Part print with two shaded views. Sizes in mm from the minimum x, y, z corner. A direction names the side the tool comes from. Give positions to 0.01 mm unless a question says otherwise; leave off trailing zeros. Write each loop counter-clockwise with the first axis right and the second up, starting at its lowest first coordinate (ties: lowest second). Pieces come first, ordered by that corner, then holes.
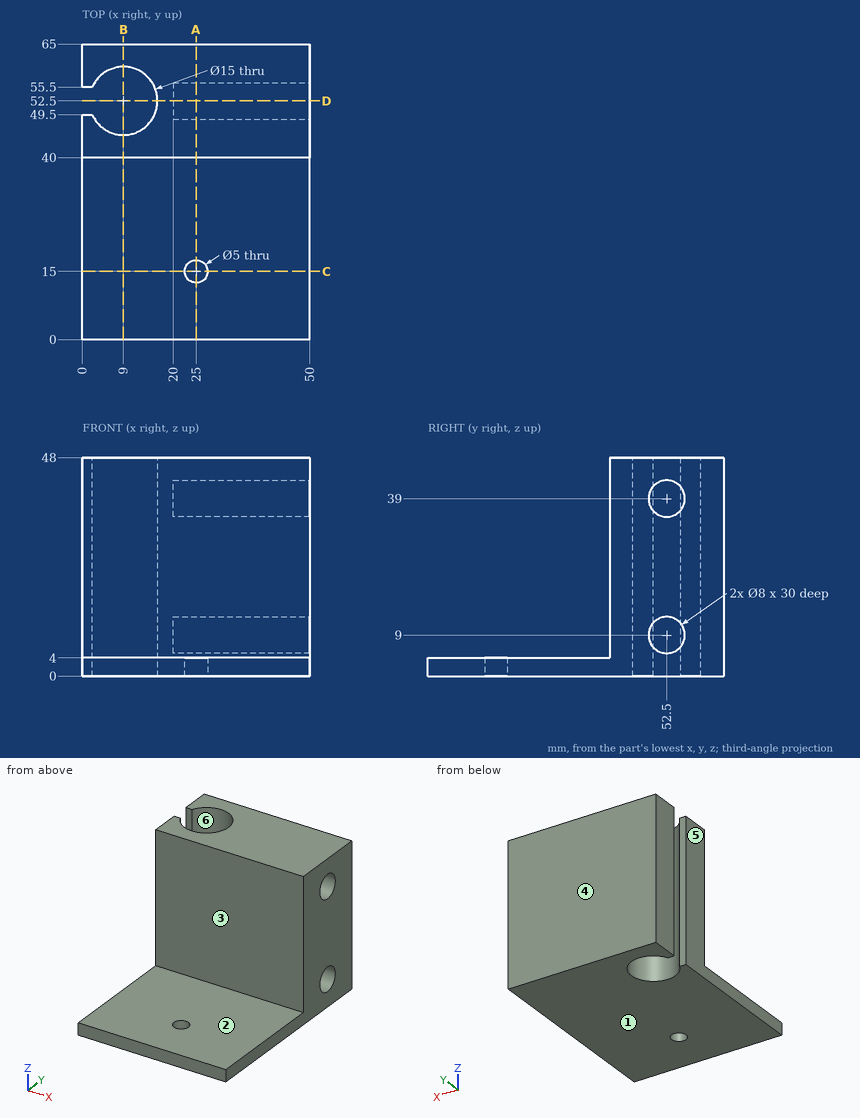
1) Mould opens along Y. For the marked faces 3, 4, 5 and 6 say: +Y half, -Y half, draft (parallel to the pull), parting line (faces both ways), or undercut.
Check result:
face 3: -Y half
face 4: +Y half
face 5: draft
face 6: undercut
2) Saw through at B-B (x = 9). Write the cut outline in (y, z), and give its area (3 significant figures).
Check result:
outline: (0, 0) - (45, 0) - (45, 48) - (40, 48) - (40, 4) - (0, 4) - close; (60, 0) - (65, 0) - (65, 48) - (60, 48) - close
area: 640 mm2
3) Saw through at A-A (x = 25). Write the cut outline in (y, z).
Check result:
outline: (0, 0) - (12.5, 0) - (12.5, 4) - (0, 4) - close; (17.5, 0) - (65, 0) - (65, 48) - (40, 48) - (40, 4) - (17.5, 4) - close; hole circle Ø8 at (52.5, 9); hole circle Ø8 at (52.5, 39)
4) 3-axis set-ups, long thin cutter, end or side, ignore diameter. For the marked faces 1 and 2: which of +Z, -Z, +X, -X, +Y, -Y reach the whole face in a straight line?
Check result:
face 1: -Z, +X, -X, +Y, -Y
face 2: +Z, +X, -X, -Y
5) Saw through at D-D (y = 52.5). Write the cut outline in (x, z), and give its area (3 significant figures).
Check result:
outline: (16.5, 0) - (50, 0) - (50, 5) - (20, 5) - (20, 13) - (50, 13) - (50, 35) - (20, 35) - (20, 43) - (50, 43) - (50, 48) - (16.5, 48) - close
area: 1,130 mm2
6) Drill centre lines: L1, parallel to Y at x = 9, z = 19; L2, parallel to Y at x = 32, z = 9; L3, parallel to Z at x = 31, y = 15.5. Where is each one in solid material? Low to high.
Check result:
L1: y = 40 to 45, 60 to 65
L2: y = 40 to 48.5, 56.5 to 65
L3: z = 0 to 4
7) Saw through at C-C (y = 15). Write the cut outline in (x, z).
Check result:
outline: (0, 0) - (22.5, 0) - (22.5, 4) - (0, 4) - close; (27.5, 0) - (50, 0) - (50, 4) - (27.5, 4) - close
8) Flat gauge pins, fed straight in: P1, Ø7, axis at y = 52.5, z = 9, coming from the +X side; P2, Ø0.6, axis at x = 1, z = 21.5, coming from the -Y side. Where does each tip first touch, or does it go through?
Check result:
P1: stops at x = 20
P2: stops at y = 40
